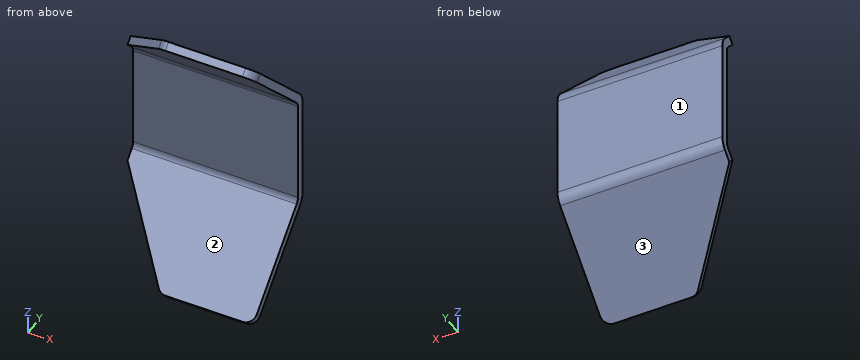
```python
from build123d import *

# Parameters (mm, degrees)
SM_BASE_FLANGE_1_DEPTH = 160
CUT_EXTRUDE_START      = 3.884627654
CUT_EXTRUDE_1_DEPTH    = 98.974499311
FILLET_1_R             = 10


# Read off the part's stored shape, not the designer's step: 切除-拉伸1
# Sheet-metal steps are written as plain solids
with BuildPart() as part:
    # Sketch 1 → 基体-法兰1 (new body)
    with BuildSketch(Plane(origin=(0, 0, 0), x_dir=(0, 0, -1), z_dir=(1, 0, 0))):
        with BuildLine():
            Line((-132.5, -80), (-54.843145751, -2.343145751))
            ThreePointArc((-54.843145751, -2.343145751), (-52.24775896, -0.60896374), (-49.186291501, 0))
            Line((-49.186291501, 0), (49.186291501, 0))
            ThreePointArc((49.186291501, 0), (52.24775896, -0.60896374), (54.843145751, -2.343145751))
            Line((54.843145751, -2.343145751), (132.5, -80))
            Line((132.5, -80), (138.156854249, -74.343145751))
            Line((138.156854249, -74.343145751), (60.5, 3.313708499))
            ThreePointArc((60.5, 3.313708499), (55.309226419, 6.78207252), (49.186291501, 8))
            Line((49.186291501, 8), (-49.186291501, 8))
            ThreePointArc((-49.186291501, 8), (-55.309226419, 6.78207252), (-60.5, 3.313708499))
            Line((-60.5, 3.313708499), (-138.156854249, -74.343145751))
            Line((-138.156854249, -74.343145751), (-132.5, -80))
        make_face()
    extrude(amount=SM_BASE_FLANGE_1_DEPTH)

    # 切除-拉伸1 outline → 切除-拉伸1 (cut)
    with BuildSketch(Plane(origin=(0, 0, 0), x_dir=(0.8944271909999176, 0.4472135954999543, 0), z_dir=(0.4472135954999544, -0.8944271909999175, 0)).offset(CUT_EXTRUDE_START)):
        Polygon((-32.422985674, 0), (-4.472135955, 62.5), (29.362637858, 138.156854249), (30.186917696, 140), (-36, 140), (-36, 7.99844719), align=None)
        Polygon((-4.472135955, -62.5), (-32.422985674, 0), (-36, -7.99844719), (-36, -140), (30.186917696, -140), (29.362637858, -138.156854249), align=None)
    extrude(amount=CUT_EXTRUDE_1_DEPTH, mode=Mode.SUBTRACT)

    # 圆角1
    fillet_1_edges = [part.edges().sort_by_distance(p)[0] for p in [
        (160, -77.171572875, -135.328427125),
        (70, -77.171572875, 135.328427125),
        (70, -77.171572875, -135.328427125),
        (160, -77.171572875, 135.328427125),
    ]]
    fillet(fillet_1_edges, radius=FILLET_1_R)


solid = part.part
```
The listing builds one solid part. Answer for the finished solid, in the listing's coordinates (mm). Face numbers are marked on the shaded views. Coordinates: 2 decimals unless noted, no trailing zeros. Loops run counter-clockwise (first coordinate to the right, second up) from the corner with the lowest first, then second, coordinate; pieces in that order, holes last. Notation, with made-up numbers: (-7.5, 50) - (16.5, 50) arc R25 cw to (16.5, 82) - close; hole circle Ø3 at (0, -16). An arc over 180 degrees is marked (long way). Write item = value, one per line.
1) Section B-B (y = -36.5) is taken. Determine the outline of the cut face in (x, z).
Responses:
outline = (26.5, -89) - (32.16, -100.31) - (160, -100.31) - (160, -89) - close; (26.5, 89) - (160, 89) - (160, 100.31) - (32.16, 100.31) - close
2) Each of these flat-tipped pins is pushed along its axis until it touches: P1, Ø8, axis at x = 93, y = -28.5, coming from the +Z side; P2, Ø3, axis at x = 107, z = 74, coming from the -Y side; P3, Ø4, axis at x = 55.5, y = -26.5, coming from the -Z side. Where does it stop, or does it pass through?
Responses:
P1 = 96.31
P2 = -23
P3 = -92.31
3) Section C-C (z = -26) is taken. Determine the outline of the cut face in (x, y), plus the area to 3 significant figures.
Responses:
outline = (0, 0) - (160, 0) - (160, 8) - (0, 8) - close
area = 1,280 mm^2
4) Section D-D (y = -52) is taken. Determine the outline of the cut face in (x, z), plus the area to 3 significant figures.
Responses:
outline = (42, -104.5) - (47.66, -115.81) - (160, -115.81) - (160, -104.5) - close; (42, 104.5) - (160, 104.5) - (160, 115.81) - (47.66, 115.81) - close
area = 2,610 mm^2
5) Determine the mould class of the marked faces 1, 2 and 3 for opening direction Z: pulls with the +Z half, pulls with the -Z half, needs draft (parallel to the pull), parting line crosses it, or undercut.
Responses:
face_1 = needs draft
face_2 = undercut
face_3 = pulls with the -Z half
6) Section A-A (x = 142.5) is taken. Determine the outline of the cut face in (y, z).
Responses:
outline = (-80, -132.5) - (-74.34, -138.16) - (3.31, -60.5) arc R16 ccw to (8, -49.19) - (8, 49.19) arc R16 ccw to (3.31, 60.5) - (-74.34, 138.16) - (-80, 132.5) - (-2.34, 54.84) arc R8 cw to (0, 49.19) - (0, -49.19) arc R8 cw to (-2.34, -54.84) - close
7) Find the intervals of material crossed by line 1 along Y through (x, z) = (24.5, 47.5); line 2 along Z through (x, y) = (60, -47); line 3 along Z through (x, y) = (24, -21), in increasing order.
Responses:
line_1 = 0 to 8
line_2 = -110.81 to -99.5, 99.5 to 110.81
line_3 = -84.81 to -73.5, 73.5 to 84.81
